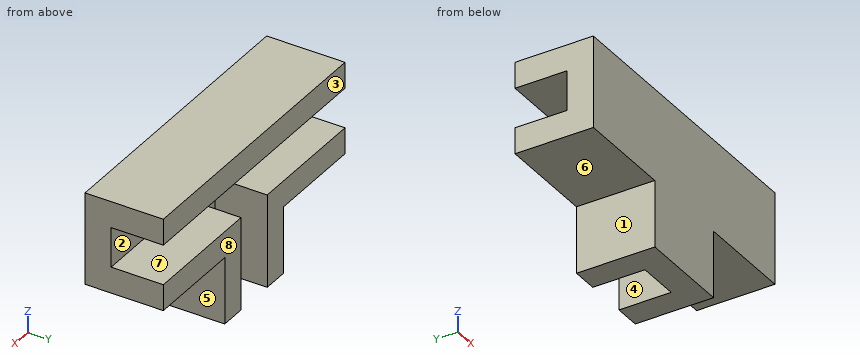
```python
from build123d import *

# Parameters (mm, degrees)
F0_W     = 27.871466
F0_H     = 5
F1_DEPTH = 15
F2_DEPTH = 10


with BuildPart() as f1:
    # F0 (on Front) → F1 (new body)
    with BuildSketch(Plane.XZ):
        Polygon((-4.015, -21.636724), (0, -21.636724), (0, 0), (0, 3.805), (-27.871466, 3.805), (-27.871466, 0), (-27.871466, -3.825), (-4.015, -3.825), align=None)
        Polygon((-9.015, -21.636724), (-4.015, -21.636724), (-4.015, -3.825), (-27.871466, -3.825), (-27.871466, -8.825), (-9.015, -8.825), align=None)
        with Locations((-13.935733, 6.305)):
            Rectangle(F0_W, F0_H)
    extrude(amount=F1_DEPTH)

    # F0 (on Front) → F2 (cut)
    with BuildSketch(Plane.XZ):
        Polygon((-4.015, -21.636724), (0, -21.636724), (0, 0), (0, 3.805), (-27.871466, 3.805), (-27.871466, 0), (-27.871466, -3.825), (-4.015, -3.825), align=None)
    extrude(amount=F2_DEPTH, mode=Mode.SUBTRACT)

    # F3: F1 across plane


with BuildPart() as f1_1:
    add(f1.part)
    add(f1.part.mirror(Plane.YZ))


solid = f1_1.part
```
Could you check a few things on this model? Use its own coordinates, in mm. Face numbers are marked on the shaded views. A direction names the side the tool comes from. Give positions to 0.01 mm unless a question says otherwise; leave off trailing zeros. Write each loop counter-clockwise with the first axis right and the second up, starting at its lowest first coordinate (ties: lowest second). Pieces come first, ordered by that corner, then holes. Notation, with made-up numbers: (68.25, -22.75) - (116.25, -22.75) arc R8 ccw to (116.25, -9.75) - close; hole circle Ø9 at (9.25, 12). An arc over 180 degrees is marked (long way). One line per item, written item: value. Start each with the question number.
Item 1: Imagine slicing it at A-A, the plane y = -3.75. List the corners of the cut face in (x, z) for me (3 decimals), and give its area (3 significant figures).
Item 2: Imagine slicing it at C-C, the plane x = -17. List the corners of the cut face in (y, z) for me (3 decimals).
Item 3: If we mould it in two halves opening along X, with no side actions, what happens to the marked faces 1, 2 and 3? For each: +X half, -X half, draft (parallel to the pull), parting line (faces both ways), or undercut.
Item 4: Please list where these lines run through material, in increasing order: line 1 (Z direction, x = 13, y = -8.5) (3 decimals); line 2 (X direction, y = -9.75, z = -14) (3 decimals); line 3 (Z direction, x = -4.5, y = -9.75) (3 decimals). Write a range as from..to.
Item 5: Imagine slicing it at B-B, the plane z = -12. List the corners of the cut face in (x, y) for me (3 decimals), and give its area (3 significant figures).
Item 6: Which directions (+Z, -Z, +X, -X, +Y, -Y) give clear straight access to the entire face, cutting with the end or side of a thin tool? Please do the marked faces 4, 5, 6, 7 and 8.
Item 7: I'm going to push flat-ended pins straight in: pin 1 (4 mm diameter, centred on y = -7, z = -12.5, fed in from +X) (3 decimals); pin 2 (5 mm diameter, centred on y = -4, z = -14, fed in from -X) (3 decimals). Where does each tip first touch, or does it pass through?
Item 8: Imagine slicing it at D-D, the plane z = 2. List the corners of the cut face in (x, y) for me, and give its area (3 significant figures).
Geometry says:
1. outline: (-27.871, -8.825) - (-9.015, -8.825) - (-9.015, -21.637) - (-4.015, -21.637) - (-4.015, -3.825) - (-27.871, -3.825) - close; (-27.871, 3.805) - (27.871, 3.805) - (27.871, 8.805) - (-27.871, 8.805) - close; (4.015, -21.637) - (9.015, -21.637) - (9.015, -8.825) - (27.871, -8.825) - (27.871, -3.825) - (4.015, -3.825) - close
1. area: 645 mm^2
2. outline: (-15, -8.825) - (0, -8.825) - (0, -3.825) - (-10, -3.825) - (-10, 3.805) - (0, 3.805) - (0, 8.805) - (-15, 8.805) - close
3. face 1: -X half
3. face 2: undercut
3. face 3: draft
4. line 1: -8.825..-3.825, 3.805..8.805
4. line 2: -9.015..-4.015, 4.015..9.015
4. line 3: -21.637..-3.825, 3.805..8.805
5. outline: (-9.015, -15) - (9.015, -15) - (9.015, 0) - (4.015, 0) - (4.015, -10) - (-4.015, -10) - (-4.015, 0) - (-9.015, 0) - close
5. area: 190 mm^2
6. face 4: -Z, +Y
6. face 5: -Z, +X, +Y, -Y
6. face 6: -Z, -X, +Y, -Y
6. face 7: +X, -X, +Y
6. face 8: +Z, -Z, +X, -X, +Y
7. pin 1: x = 9.015
7. pin 2: x = -9.015
8. outline: (-27.87, -15) - (27.87, -15) - (27.87, -10) - (-27.87, -10) - close
8. area: 279 mm^2
